Model file for the job. Use its own axes, mm. A direction names the side the tool comes from. Coordinates: 2 decimals unless noted, no trailing zeros. Write each loop counter-clockwise with the first axis right and the second up, starting at its lowest first coordinate (ties: lowest second). Pieces come first, ordered by that corner, then holes. Notation, with made-up numbers: M 82.25,-29.75 L 130.25,-29.75 A37 cw 130.25,8.25 Z; hole C 15,86 d1. An arc over 180 degrees is marked long. Put each result on its own line as item: value. Start each with the question number.
Q1. Cut at A-A (y = -25). Write the cut outline in (x, z), then the cut area to 3 significant figures.
Q2. Drop flat-ended pins along their axis: pin 1 (3 mm diameter, centred on y = -17, z = 1, fed in from -X); pin 2 (1.7 mm diameter, centred on x = -0.99, z = 5.5, fed in from -Y); pin 3 (1.5 mm diameter, centred on x = -1.5, y = -22, fed in from -Z). Give the stop position or say it passes through.
Q3. Drill centre lines: line 1 along X through (y, z) = (3.5, -5.5); line 2 along X through (y, z) = (3.25, 9.5); line 3 along Y through (x, z) = (8, -4.75). Where is each one in solid material? Low to high.
Q4. Pull direction X, two halves, no side cores. Call faces 3 (the cylindrical face through (-10.74, 3.51, -2.38)), 4 (the cylindrical face through (0.04, 3.37, 8.75)), 5 (the flat face through (3, 4, -3)): pulls with the +X half, pulls with the -X half, needs draft (parallel to the pull), parting line crosses it, or undercut.
Q5. Which spindle directions (+Z, -Z, +X, -X, +Y, -Y) get a long thin tool onto all of the face, cutting with end or side? Do faces 1 (the cylindrical face through (-1, -13, 0)), 2 (the cylindrical face through (-4.857, 3.134, -0.597)). Say none if no direction does.
```python
from build123d import *

# Parameters (mm, degrees)
SKETCH2_R          = 0.75
SKETCH2_R_2        = 0.5
CUT_EXTRUDE1_DEPTH = 40


with BuildPart() as part:
    # Sketch1 → Revolve1 (revolve)
    with BuildSketch(Plane(origin=(0, 0, 0), x_dir=(0, 0, -1), z_dir=(1, 0, 0))):
        with BuildLine():
            ThreePointArc((-3.5, 4), (-2.474873734, 1.525126266), (0, 0.5))
            Line((0, 0.5), (0, 0))
            Line((0, 0), (0, -25.34))
            Line((0, -25.34), (0, -31.34))
            ThreePointArc((0, -31.34), (-2.956795679, -28.847305936), (-1, -25.511572875))
            Line((-1, -25.511572875), (-1, 0.127016654))
            ThreePointArc((-1, 0.127016654), (-2.457034335, 0.843580783), (-3.50920881, 2.080246493))
            Line((-3.50920881, 2.080246493), (-11, 3))
            Line((-11, 3), (-11, 4))
            Line((-11, 4), (-4, 4))
            Line((-4, 4), (-3.5, 4))
        make_face()
    revolve(axis=Axis((0, 10.634252877, 0), (0, 1, 0)))

    # Sketch2 → Cut-Extrude1 (cut)
    with BuildSketch(Plane(origin=(0, 4, 0), x_dir=(1, 0, 0), z_dir=(0, 1, 0))):
        with Locations(Location((-5.489872585, -1, 0), (0, 0, 270))):
            Circle(SKETCH2_R)
        with Locations(Location((-9.5, 0, 0), (0, 0, 270))):
            Circle(SKETCH2_R)
        with Locations(Location((0.00965171, -9.5, 0), (0, 0, 270))):
            Circle(SKETCH2_R)
        with Locations(Location((-0.990356221, -5.500003966, 0), (0, 0, 270))):
            Circle(SKETCH2_R)
        with Locations(Location((1.009643779, -5.5, 0), (0, 0, 270))):
            Circle(SKETCH2_R)
        with Locations(Location((5.509142299, -0.999978192, 0), (0, 0, 270))):
            Circle(SKETCH2_R)
        with Locations(Location((5.509134368, 1.000021808, 0), (0, 0, 270))):
            Circle(SKETCH2_R)
        with Locations(Location((9.519265749, 3.7711e-05, 0), (0, 0, 270))):
            Circle(SKETCH2_R)
        with Locations(Location((1.009643779, 5.5, 0), (0, 0, 270))):
            Circle(SKETCH2_R)
        with Locations(Location((-0.990356221, 5.500003966, 0), (0, 0, 270))):
            Circle(SKETCH2_R)
        with Locations(Location((0.00965171, 9.5, 0), (0, 0, 270))):
            Circle(SKETCH2_R)
        with Locations(Location((0, 0, 0), (0, 0, 270))):
            Circle(SKETCH2_R_2)
        with Locations(Location((-5.489872585, 1, 0), (0, 0, 270))):
            Circle(SKETCH2_R)
    extrude(amount=-CUT_EXTRUDE1_DEPTH, mode=Mode.SUBTRACT)


solid = part.part
```
Computed values:
1. outline: C 0,0 d2; hole C 0,0 d1
1. area: 2.36 mm2
2. pin 1: x = -1
2. pin 2: y = 2.23
2. pin 3: z = -0.66
3. line 1: -9.53 to -1.74, -0.24 to 0.26, 1.76 to 9.53
3. line 2: -5.55 to -0.74, 0.76 to 5.55
3. line 3: 2.79 to 4
4. face 3: parting line crosses it
4. face 4: undercut
4. face 5: needs draft
5. face 1: none
5. face 2: +Y, -Y
